```python
from build123d import *

# Parameters (mm, degrees)
F0_W     = 120
F0_H     = 114
F1_DEPTH = 3
F2_W     = 20
F2_H     = 2.5
F3_DEPTH = 5
F4_R     = 4.99999
F5_R     = 1.5
F6_W     = 5
F6_H     = 7.5
F7_DEPTH = 25


# Not quite as in the source:
# - a fillet or chamfer is up to 0.001 mm smaller than in the source, because OpenCascade refuses the exact size


with BuildPart() as f1:
    # F0 (on Front) → F1 (new body)
    with BuildSketch(Plane.XZ):
        with Locations((60, 57)):
            Rectangle(F0_W, F0_H)
    extrude(amount=F1_DEPTH)

    # F2 (on face) → F3 (join)
    with BuildSketch(Plane.XZ.offset(3)):
        with Locations((10, 112.75)):
            Rectangle(F2_W, F2_H)
        with Locations((110, 112.75)):
            Rectangle(F2_W, F2_H)
    extrude(amount=F3_DEPTH)

    # F4 (radius 5 in the source; OpenCascade refuses exactly that, so slightly less here)
    f4_edges = [f1.edges().sort_by_distance(p)[0] for p in [
        (20, -8, 112.75),
        (100, -8, 112.75),
    ]]
    fillet(f4_edges, radius=F4_R)

    # F5
    f5_edges = [f1.edges().sort_by_distance(p)[0] for p in [
        (7.500005, -8, 114),
        (112.499995, -8, 114),
    ]]
    fillet(f5_edges, radius=F5_R)

    # F6 (on face) → F7 (cut)
    with BuildSketch(Plane(origin=(0, 0, 0), x_dir=(-1, 0, 0), z_dir=(0, 1, 0))):
        with Locations((-117.5, 3.75)):
            Rectangle(F6_W, F6_H)
    extrude(amount=-F7_DEPTH, mode=Mode.SUBTRACT)


solid = f1.part
```
Geometry: final body of the model. Coordinates: model frame, mm. A direction names the side the tool comes from. Give positions to 0.01 mm unless a question says otherwise; leave off trailing zeros. Loops run counter-clockwise (first coordinate to the right, second up) from the corner with the lowest first, then second, coordinate; pieces in that order, holes last. Notation, with made-up numbers: (64.25, 27) -> (73.25, 27) arc R11 ccw to (73.25, 37) -> close; hole circle Ø10 at (23, -24). An arc over 180 degrees is marked (long way). Use CSV: the item, a comma, the result in double quotes.
(1) Pull-direction query (X, two-part tool) for faces 1 (the face through (59, 0, 58)), 2 (the face through (0, -2, 61)), 3 (the face through (102, -7, 112)); classes: released by +X, released by -X, zero draft, split by the parting line, or undercut.
From the geometry:
face 1,"zero draft"
face 2,"released by -X"
face 3,"undercut"
(2) Ray query, line 1 along Y through (x, z) = (61.5, 62.5); line 2 along Z through (x, y) = (13.5, -6); line 3 along X through (y, z) = (-0.5, 7). Return the intervals inside material, ascending. Write a range as [from, to].
From the geometry:
line 1,"[-3, 0]"
line 2,"[111.5, 114]"
line 3,"[0, 115]"
(3) First-contact query: P1, Ø1.5, axis at y = -1.5, z = 4, coming from the +X side; P2, Ø2, axis at x = 95, z = 22.5, coming from the -Y side; P3, Ø1.5, axis at x = 114, y = -5.5, coming from the -Z side; P4, Ø1.5, axis at y = -3, z = 90.5, coming from the -X side. Flat tips, straight axial feed; report the tip coordinate or a pass-through.
From the geometry:
P1,"x = 115"
P2,"y = -3"
P3,"z = 111.5"
P4,"x = 0"
(4) Cut plane B-B (x = 66). Output: boundary loops of the cut face in (y, z).
From the geometry:
outline,"(-3, 0) -> (0, 0) -> (0, 114) -> (-3, 114) -> close"
(5) Access query for faces 4 (the face through (118, -1, 7.5)), 5 (the face through (19, -6, 112)), 6 (the face through (110, -5, 111.5)). Directions: +Z, -Z, +X, -X, +Y, -Y. A direction counts if a zero-diameter tool reaches every point of the face in a straight line with its end or side. Return the directions, or none.
From the geometry:
face 4,"-Z, +X, +Y, -Y"
face 5,"+Z, -Z, -Y"
face 6,"-Z, +X, -X, -Y"
(6) Cut plane A-A (z = 58). Output: boundary loops of the cut face in (x, y).
From the geometry:
outline,"(0, -3) -> (120, -3) -> (120, 0) -> (0, 0) -> close"
